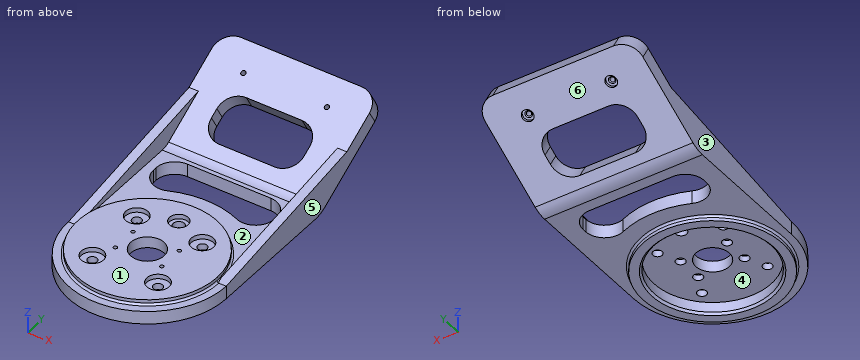
from build123d import *

# Parameters (mm, degrees)
SKETCH_1_R            = 37.5
EXTRUDE_1_DEPTH       = 12.5
SKETCH_2_R            = 31.6
CUT_EXTRUDE_1_DEPTH   = 6.5
CUT_EXTRUDE_2_REACH   = 56.486
SKETCH_3_R            = 2.5
SKETCH_4_R            = 6
CUT_EXTRUDE_3_DEPTH   = 2.5
CHAMFER_2_SIZE        = 1.1
SKETCH_14_R           = 1.025
CUT_EXTRUDE_4_DEPTH   = 6
SKETCH_15_R           = 2.5
CUT_EXTRUDE_5_DEPTH   = 3
SKETCH_17_R           = 9
CUT_EXTRUDE_7_DEPTH   = 6
SKETCH_18_R           = 3
CUT_EXTRUDE_8_DEPTH   = 6
SKETCH_19_R           = 5
CUT_EXTRUDE_9_DEPTH   = 2.5
SKETCH_24_R           = 42.5
SKETCH_24_R_2         = 37.5
EXTRUDE_2_DEPTH       = 3.5
EXTRUDE_START         = 40.640001537
EXTRUDE_3_OUTLINE_W   = 132.359796054
EXTRUDE_3_OUTLINE_H   = 7
EXTRUDE_3_DEPTH       = 34.359998463
EXTRUDE_START_2       = 2.75
EXTRUDE_3_2_DEPTH     = 7
EXTRUDE_START_3       = 26.556252313
EXTRUDE_3_3_OUTLINE_W = 132.359796054
EXTRUDE_3_3_OUTLINE_H = 60
EXTRUDE_3_3_DEPTH     = 8.562177827
EXTRUDE_3_4_OUTLINE_W = 132.359796054
EXTRUDE_3_4_OUTLINE_H = 0.830127019
EXTRUDE_3_4_DEPTH     = 2.5
CUT_EXTRUDE_11_DEPTH  = 47.359796
CUT_EXTRUDE_12_DEPTH  = 7
RIB_10_REACH          = 159.979
SKETCH_31_WALL_W      = 415.104412192
SKETCH_31_WALL_H      = 5
FILLET_6_R            = 10
FILLET_7_R            = 10
SKETCH_34_R           = 1.25
CUT_EXTRUDE_14_DEPTH  = 8.562177826
SKETCH_35_R           = 3
CUT_EXTRUDE_15_DEPTH  = 1.5
CUT_EXTRUDE_16_DEPTH  = 8.562177826
FILLET_9_R            = 1
FILLET_10_R           = 15
CHAMFER_3_SIZE        = 0.5
FILLET_11_R           = 10
FILLET_12_R           = 10


with BuildPart() as part:
    # 草图1 → 凸台-拉伸1 (new body)
    with BuildSketch(Plane.XY):
        Circle(SKETCH_1_R)
    extrude(amount=EXTRUDE_1_DEPTH)

    # 草图2 → 切除-拉伸1 (cut)
    with BuildSketch(Plane(origin=(0, 0, 0), x_dir=(-1, 0, 0), z_dir=(0, 0, -1))):
        Circle(SKETCH_2_R)
    extrude(amount=-CUT_EXTRUDE_1_DEPTH, mode=Mode.SUBTRACT)

    # 草图3 → 切除-拉伸2 (cut, up to next)
    with BuildSketch(Plane.XY.offset(12.5), mode=Mode.PRIVATE) as cut_extrude_2_sk1:
        with Locations((17.67766953, 17.67766953)):
            Circle(SKETCH_3_R)
    cut_extrude_2_tool1 = extrude(cut_extrude_2_sk1.sketch, amount=-CUT_EXTRUDE_2_REACH, mode=Mode.PRIVATE) & part.part
    # 草图3 → 切除-拉伸2 (cut, up to next)
    with BuildSketch(Plane.XY.offset(12.5), mode=Mode.PRIVATE) as cut_extrude_2_sk2:
        with Locations(Location((17.67766953, -17.67766953, 0), (0, 0, 180))):
            Circle(SKETCH_3_R)
    cut_extrude_2_tool2 = extrude(cut_extrude_2_sk2.sketch, amount=-CUT_EXTRUDE_2_REACH, mode=Mode.PRIVATE) & part.part
    # 草图3 → 切除-拉伸2 (cut, up to next)
    with BuildSketch(Plane.XY.offset(12.5), mode=Mode.PRIVATE) as cut_extrude_2_sk3:
        with Locations((-17.67766953, -17.67766953)):
            Circle(SKETCH_3_R)
    cut_extrude_2_tool3 = extrude(cut_extrude_2_sk3.sketch, amount=-CUT_EXTRUDE_2_REACH, mode=Mode.PRIVATE) & part.part
    # 草图3 → 切除-拉伸2 (cut, up to next)
    with BuildSketch(Plane.XY.offset(12.5), mode=Mode.PRIVATE) as cut_extrude_2_sk4:
        with Locations(Location((-17.67766953, 17.67766953, 0), (0, 0, 180))):
            Circle(SKETCH_3_R)
    cut_extrude_2_tool4 = extrude(cut_extrude_2_sk4.sketch, amount=-CUT_EXTRUDE_2_REACH, mode=Mode.PRIVATE) & part.part
    add(cut_extrude_2_tool1.solids().sort_by_distance((17.67767, 17.67767, 12.5))[0], mode=Mode.SUBTRACT)
    add(cut_extrude_2_tool2.solids().sort_by_distance((17.67767, -17.67767, 12.5))[0], mode=Mode.SUBTRACT)
    add(cut_extrude_2_tool3.solids().sort_by_distance((-17.67767, -17.67767, 12.5))[0], mode=Mode.SUBTRACT)
    add(cut_extrude_2_tool4.solids().sort_by_distance((-17.67767, 17.67767, 12.5))[0], mode=Mode.SUBTRACT)

    # 草图4 → 切除-拉伸3 (cut)
    with BuildSketch(Plane.XY.offset(12.5)):
        with Locations((-17.67766953, 17.67766953)):
            Circle(SKETCH_4_R)
        with Locations(Location((17.67766953, 17.67766953, 0), (0, 0, 180))):
            Circle(SKETCH_4_R)
        with Locations((17.67766953, -17.67766953)):
            Circle(SKETCH_4_R)
        with Locations(Location((-17.67766953, -17.67766953, 0), (0, 0, 180))):
            Circle(SKETCH_4_R)
    extrude(amount=-CUT_EXTRUDE_3_DEPTH, mode=Mode.SUBTRACT)

    # 倒角2
    chamfer_2_edges = [part.edges().sort_by_distance(p)[0] for p in [
        (31.6, 0, 0),
    ]]
    chamfer(chamfer_2_edges, length=CHAMFER_2_SIZE)

    # 草图14 → 切除-拉伸4 (cut)
    with BuildSketch(Plane(origin=(0, 0, 6.5), x_dir=(-1, 0, 0), z_dir=(0, 0, -1))):
        with Locations((12.5, 7)):
            Circle(SKETCH_14_R)
        with Locations(Location((12.5, -7, 0), (0, 0, 180))):
            Circle(SKETCH_14_R)
        with Locations((-12.5, -7)):
            Circle(SKETCH_14_R)
        with Locations(Location((-12.5, 7, 0), (0, 0, 180))):
            Circle(SKETCH_14_R)
    extrude(amount=-CUT_EXTRUDE_4_DEPTH, mode=Mode.SUBTRACT)

    # 草图15 → 切除-拉伸5 (cut)
    with BuildSketch(Plane(origin=(0, 0, 6.5), x_dir=(-1, 0, 0), z_dir=(0, 0, -1))):
        with Locations((12.5, 7)):
            Circle(SKETCH_15_R)
        with Locations((12.5, -7)):
            Circle(SKETCH_15_R)
        with Locations((-12.5, -7)):
            Circle(SKETCH_15_R)
        with Locations((-12.5, 7)):
            Circle(SKETCH_15_R)
    extrude(amount=-CUT_EXTRUDE_5_DEPTH, mode=Mode.SUBTRACT)

    # 草图17 → 切除-拉伸7 (cut)
    with BuildSketch(Plane.XY.offset(12.5)):
        Circle(SKETCH_17_R)
    extrude(amount=-CUT_EXTRUDE_7_DEPTH, mode=Mode.SUBTRACT)

    # 草图18 → 切除-拉伸8 (cut)
    with BuildSketch(Plane.XY.offset(12.5)):
        with Locations((0, 25)):
            Circle(SKETCH_18_R)
    extrude(amount=-CUT_EXTRUDE_8_DEPTH, mode=Mode.SUBTRACT)

    # 草图19 → 切除-拉伸9 (cut)
    with BuildSketch(Plane.XY.offset(12.5)):
        with Locations((0, 25)):
            Circle(SKETCH_19_R)
    extrude(amount=-CUT_EXTRUDE_9_DEPTH, mode=Mode.SUBTRACT)

    # 草图24 → 凸台-拉伸2 (add, symmetric)
    with BuildSketch(Plane(origin=(0, 0, 6.25), x_dir=(-1, 0, 0), z_dir=(0, 0, -1))):
        Circle(SKETCH_24_R)
        Circle(SKETCH_24_R_2, mode=Mode.SUBTRACT)
    extrude(amount=EXTRUDE_2_DEPTH, both=True)

    # 凸台-拉伸3: read off the stored shape, not the designer's step
    # 凸台-拉伸3 outline → 凸台-拉伸3 (add)
    with BuildSketch(Plane(origin=(0, 0, 0), x_dir=(1, 0, 0), z_dir=(0, 1, 0)).offset(EXTRUDE_START)):
        with Locations((-23.679898027, -6.25)):
            Rectangle(EXTRUDE_3_OUTLINE_W, EXTRUDE_3_OUTLINE_H)
    extrude(amount=EXTRUDE_3_DEPTH)

    # Extrude 3 2 outline → Extrude 3 2 (add)
    with BuildSketch(Plane.XY.offset(EXTRUDE_START_2)):
        with BuildLine():
            Line((-89.859796054, 40.640001537), (-89.859796054, 0))
            Line((-89.859796054, 0), (-42.5, 0))
            ThreePointArc((-42.5, 0), (-34.166916622, 25.275913604), (-12.435444305, 40.640001537))
            Line((-12.435444305, 40.640001537), (-89.859796054, 40.640001537))
        make_face()
        with BuildLine():
            ThreePointArc((12.435444305, 40.640001537), (34.166916622, 25.275913604), (42.5, 0))
            Line((42.5, 0), (42.5, 40.640001537))
            Line((42.5, 40.640001537), (12.435444305, 40.640001537))
        make_face()
    extrude(amount=EXTRUDE_3_2_DEPTH)

    # Extrude 3 3 outline → Extrude 3 3 (add)
    with BuildSketch(Plane(origin=(0, 0, 0), x_dir=(1, 0, 0), z_dir=(0, 0.500000000000001, -0.866025403784438)).offset(EXTRUDE_START_3)):
        with Locations((-23.679898027, -96.326905284)):
            Rectangle(EXTRUDE_3_3_OUTLINE_W, EXTRUDE_3_3_OUTLINE_H)
    extrude(amount=EXTRUDE_3_3_DEPTH)

    # Extrude 3 4 outline → Extrude 3 4 (add)
    with BuildSketch(Plane(origin=(0, 0, 0), x_dir=(1, 0, 0), z_dir=(0, 0.500000000000001, -0.866025403784438)).offset(EXTRUDE_START_3)):
        with Locations((-23.679898027, -65.911841775)):
            Rectangle(EXTRUDE_3_4_OUTLINE_W, EXTRUDE_3_4_OUTLINE_H)
    extrude(amount=EXTRUDE_3_4_DEPTH)

    # 草图26 → 切除-拉伸11 (cut)
    with BuildSketch(Plane.ZY.offset(89.859796054)):
        Polygon((9.75, 0), (9.75, 70), (40.165063509, 122.680435314), (32.75, 126.961524227), (2.75, 75), (2.75, 0), align=None)
    extrude(amount=-CUT_EXTRUDE_11_DEPTH, mode=Mode.SUBTRACT)

    # 草图27 → 切除-拉伸12 (cut)
    with BuildSketch(Plane(origin=(0, 0, 2.75), x_dir=(-1, 0, 0), z_dir=(0, 0, -1))):
        with BuildLine():
            Line((32.5, 34.641016151), (32.5, 65))
            Line((32.5, 65), (-32.5, 65))
            Line((-32.5, 65), (-32.5, 34.641016151))
            ThreePointArc((-32.5, 34.641016151), (0, 47.5), (32.5, 34.641016151))
        make_face()
    extrude(amount=-CUT_EXTRUDE_12_DEPTH, mode=Mode.SUBTRACT)

    # 草图31 wall → 筋10 (add, up to next)
    with BuildSketch(Plane(origin=(-42.5, 47.990381057, 17.25), x_dir=(0, -0.988007313769, -0.15440708513), z_dir=(0, -0.15440708513, 0.988007313769)), mode=Mode.PRIVATE) as rib_10_sk1:
        with Locations((0, 2.5)):
            Rectangle(SKETCH_31_WALL_W, SKETCH_31_WALL_H)
    rib_10_tool1 = extrude(rib_10_sk1.sketch, amount=-RIB_10_REACH, mode=Mode.PRIVATE) - part.part
    rib_10 = rib_10_tool1.solids().sort_by_distance((-42.5, 47.990381057, 17.25))[0]
    add(rib_10)

    # 镜向2: 筋10 across plane
    add(rib_10.mirror(Plane(origin=(0, 0, 0), x_dir=(0, 0, 1), z_dir=(1, 0, 0))))

    # 圆角6
    fillet_6_edges = [part.edges().sort_by_distance(p)[0] for p in [
        (0, 70, 9.75),
    ]]
    fillet(fillet_6_edges, radius=FILLET_6_R)

    # 圆角7
    fillet_7_edges = [part.edges().sort_by_distance(p)[0] for p in [
        (42.5, 124.820979771, 36.457531755),
        (-42.500000054, 124.82097977, 36.457531755),
    ]]
    fillet(fillet_7_edges, radius=FILLET_7_R)

    # 草图34 → 切除-拉伸14 (cut)
    with BuildSketch(Plane(origin=(0, 13.278126157, -22.998389132), x_dir=(1, 0, 0), z_dir=(0, -0.5000000000000017, 0.8660254037844378))):
        with Locations(Location((-22.5, 111.326905284, 0), (0, 0, 270))):
            Circle(SKETCH_34_R)
        with Locations(Location((22.5, 111.326905284, 0), (0, 0, 90))):
            Circle(SKETCH_34_R)
    extrude(amount=-CUT_EXTRUDE_14_DEPTH, mode=Mode.SUBTRACT)

    # 草图35 → 切除-拉伸15 (cut)
    with BuildSketch(Plane(origin=(0, 17.55921507, -30.413452642), x_dir=(-1, 0, 0), z_dir=(0, 0.5000000000000013, -0.8660254037844379))):
        with Locations(Location((-22.5, 111.326905284, 0), (0, 0, 90))):
            Circle(SKETCH_35_R)
        with Locations(Location((22.5, 111.326905284, 0), (0, 0, 90))):
            Circle(SKETCH_35_R)
    extrude(amount=-CUT_EXTRUDE_15_DEPTH, mode=Mode.SUBTRACT)

    # 草图36 → 切除-拉伸16 (cut)
    with BuildSketch(Plane(origin=(0, 13.278126157, -22.998389132), x_dir=(1, 0, 0), z_dir=(0, -0.5000000000000017, 0.8660254037844378))):
        with BuildLine():
            Line((-15, 76.176270189), (15, 76.176270189))
            ThreePointArc((15, 76.176270189), (22.071067812, 79.105202377), (25, 86.176270189))
            Line((25, 86.176270189), (25, 91.176270189))
            ThreePointArc((25, 91.176270189), (22.071067812, 98.247338001), (15, 101.176270189))
            Line((15, 101.176270189), (-15, 101.176270189))
            ThreePointArc((-15, 101.176270189), (-22.071067812, 98.247338001), (-25, 91.176270189))
            Line((-25, 91.176270189), (-25, 86.176270189))
            ThreePointArc((-25, 86.176270189), (-22.071067812, 79.105202377), (-15, 76.176270189))
        make_face()
    extrude(amount=-CUT_EXTRUDE_16_DEPTH, mode=Mode.SUBTRACT)

    # 圆角9
    # the kernel refuses this fillet: 1 mm, written as the material it adds along each edge
    with BuildSketch(Plane(origin=(0, 0, 9.75), x_dir=(-1.0, 3.747518651596283e-12, 0), z_dir=(-3.747518651596283e-12, -1.0, 0))) as fillet_9_piece_1:
        with BuildLine():
            CenterArc((37.5 + FILLET_9_R, -FILLET_9_R), FILLET_9_R, 90, 90)
            Line((37.5, -FILLET_9_R), (37.5, 0))
            Line((37.5, 0), (37.5 + FILLET_9_R, 0))
        make_face()
    revolve(axis=Axis((0, 0, 9.75), (0, 0, -1)), revolution_arc=180)
    with BuildSketch(Plane(origin=(0, 0, 2.75), x_dir=(1, 0, 0), z_dir=(0, 1, 0))) as fillet_9_piece_2:
        with BuildLine():
            CenterArc((37.5 + FILLET_9_R, FILLET_9_R), FILLET_9_R, 180, 90)
            Line((37.5, FILLET_9_R), (37.5, 0))
            Line((37.5, 0), (37.5 + FILLET_9_R, 0))
        make_face()
    revolve(axis=Axis((0, 0, 2.75), (0, 0, -1)))
    with BuildSketch(Plane(origin=(0, 0, 9.75), x_dir=(1, 0, 0), z_dir=(0, 1, 0))) as fillet_9_piece_3:
        with BuildLine():
            CenterArc((37.5 + FILLET_9_R, -FILLET_9_R), FILLET_9_R, 90, 90)
            Line((37.5, -FILLET_9_R), (37.5, 0))
            Line((37.5, 0), (37.5 + FILLET_9_R, 0))
        make_face()
    revolve(axis=Axis((0, 0, 9.75), (0, 0, -1)), revolution_arc=180)

    # 圆角10
    fillet_10_edges = [part.edges().sort_by_distance(p)[0] for p in [
        (-2.7e-08, 75, 2.75),
    ]]
    fillet(fillet_10_edges, radius=FILLET_10_R)

    # 倒角3
    chamfer_3_edges = [part.edges().sort_by_distance(p)[0] for p in [
        (22.5, 112.138611416, 25.924038106),
        (-22.5, 114.303674925, 27.174038106),
    ]]
    chamfer(chamfer_3_edges, length=CHAMFER_3_SIZE)

    # 圆角11
    fillet_11_edges = [part.edges().sort_by_distance(p)[0] for p in [
        (32.5, 65, 6.25),
        (-32.5, 65, 6.25),
    ]]
    fillet(fillet_11_edges, radius=FILLET_11_R)

    # 圆角12
    fillet_12_edges = [part.edges().sort_by_distance(p)[0] for p in [
        (-32.5, 34.641016151, 6.25),
        (32.5, 34.641016151, 6.25),
    ]]
    fillet(fillet_12_edges, radius=FILLET_12_R)


solid = part.part
The model under review builds one solid part; all positions refer to its coordinate system, in mm. Face numbers are marked on the shaded views. A direction names the side the tool comes from. Round coordinates to 2 decimals unless told otherwise and drop trailing zeros. Use one line per item in the form item = value.
Q1. Clearance check with flat-ended pins moving along their axes: P1, Ø2, axis at x = 11, y = 108.5, coming from the -Z side; P2, Ø14, axis at x = -17.68, y = -17.68, coming from the -Z side; P3, Ø4, axis at x = 24, z = 26.5, coming from the +Y side; P4, Ø1.6, axis at x = 12.5, y = -7, coming from the -Z side. State where each tip first meets the part, or that it passes through.
Response values:
P1 = 21.51
P2 = 0.7
P3 = 119.6
P4 = through
Q2. Tool access review of the marked faces 1, 2 and 3: name each direction out of +Z, -Z, +X, -X, +Y, -Y from which nothing blocks a thin tool from reaching the whole face with its end or side.
Response values:
face_1 = +Z, -Y
face_2 = +Z
face_3 = +Z, -Z, -X, +Y, -Y
Q3. Mouldability with a two-part tool opening along X and no side actions: class the marked faces 4, 5 and 6 as pulls with the +X half, pulls with the -X half, needs draft (parallel to the pull), parting line crosses it, or undercut.
Response values:
face_4 = undercut
face_5 = pulls with the +X half
face_6 = needs draft
Q4. Add section A-A on x = 17. Give the number of separate pieces and of enclosed holes in the cut face, then the cut area to 3 significant figures.
Response values:
separate_pieces = 5
enclosed_holes = 0
area = 869 mm^2
Q5. To check wall thickness, follow line 1 (Y direction, x = 0, z = 11); line 2 (X direction, y = 27.5, z = 11); line 3 (Y direction, x = -17, z = 11.5). State the ranges of each line that lie inside material, in increasing order.
Response values:
line_1 = -37.5 to -9, 9 to 20, 30 to 37.5, 72.16 to 81.61
line_2 = -42.5 to -37.5, -25.5 to -4.33, 4.33 to 25.5, 37.5 to 42.5
line_3 = -33.43 to -23.64, -11.72 to 11.72, 23.64 to 33.43, 73.03 to 81.55
